Verification items for the finished model (mm, model axes). Face numbers are marked on the shaded views. A direction names the side the tool comes from. Round coordinates to 2 decimals unless told otherwise and drop trailing zeros. Order: outer loops, then holes, each group sorted by start corner. A loop starts at its lowest first (then second) coordinate and runs counter-clockwise, first axis right, second up. Notation, with made-up numbers: (-16, 6.5) -> (31, 6.5) arc R26 cw to (31, 26.5) -> close; hole circle Ø11 at (-7, 47). An arc over 180 degrees is marked (long way). Put each result on its own line as item: value.
Autodesk Inventor part; units mm, degrees
ref_plane "YZ Plane" through (0, 0, 0) normal (1, 0, 0) x (0, 1, 0)
ref_plane "XZ Plane" through (0, 0, 0) normal (0, 1, 0) x (-1, 0, 0)
ref_plane "XY Plane" through (0, 0, 0) normal (0, 0, 1) x (1, 0, 0)
sketch "Sketch1" plane through (0, 0, 0) normal (1, 0, 0) x (0, 1, 0)
  line L0 (-11, 0) -> (11, 0)
  line L1 (13, -8.587477) -> (0, -8.587477)
  line L2 (0, -8.587477) -> (0, 9)
  line L3 (0, 9) -> (4, 9)
  line L4 (4, 9) -> (11, 0) construction
  line L5 (4, 9) -> (13, 7)
  line L6 (13, 7) -> (13, 2)
  line L7 (13, 2) -> (13, 0)
  line L8 (4, 9) -> (0, 9)
  line L9 (0, 9) -> (0, 23)
  line L10 (0, 23) -> (4, 23)
  line L11 (4, 23) -> (4, 9)
  line L12 (13, -8.587477) -> (13, 0)
  point P0 (0, 0)
  dimension "d12" = 4
  dimension "d13" = 0
  dimension "d15" = 13
  dimension "d16" = 0
  dimension "d17" = 2
  dimension "d19" = 5
  dimension "d20" = 14
revolve "Revolution1" add sketch "Sketch1" angle 360 about axis through (0, 0, -8.587477) along (0, 0, 1)
sketch "Sketch4" plane through (0, 0, 23) normal (0, 0, 1) x (1, 0, 0)
  circle A0 centre (0, 0) radius 1.479649
  circle A1 centre (0, 0) radius 4
  circle A2 centre (0, 0) radius 3.25
  point P0 (0, 0)
  dimension "d21" = 6.5
extrude "Extrusion2" cut sketch "Sketch4" against normal through all contours A0 | A2
sketch "Sketch5" plane through (0, 0, -8.587477) normal (0, 0, -1) x (-1, 0, 0)
  circle A0 centre (0, 0) radius 11.938351
  circle A1 centre (0, 0) radius 11.2
  circle A2 centre (0, 0) radius 11
  point P0 (0, 0)
  dimension "d28" = 0.2
sketch "Sketch5 outline for Extrusion3" plane through (0, 0, -8.587477) normal (0, 0, -1) x (-1, 0, 0)
  circle A0 centre (0, 0) radius 11.2
extrude "Extrusion3" cut sketch "Sketch5 outline for Extrusion3" against normal blind 12 draft -3
fillet "Fillet2" radius 2 4 edges at (0, -4, 9) (0, -13, 7) (10.5711, 0, 3.4125) (-3.25, 0, 3.4125)
properties part number "01_Connector_T"
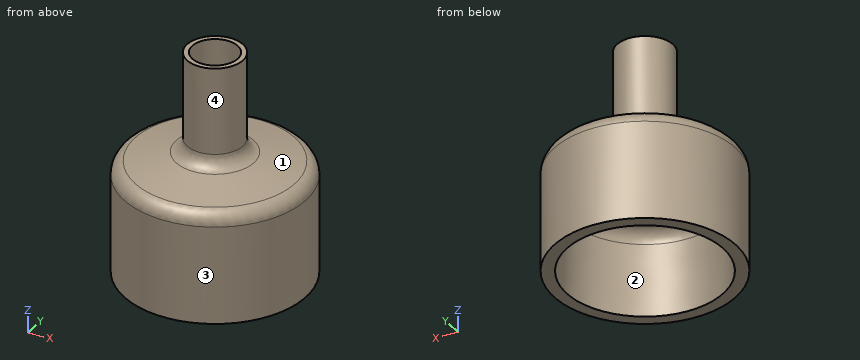
Item 1: Gauge pin test, flat ends, axial feed: pin 1 Ø8 at (x, y) = (0.5, -10) entering from -Z; pin 2 Ø4 at (x, y) = (-6, 3.5) entering from -Z; pin 3 Ø3 at (y, z) = (-2, -2) entering from -X; pin 4 Ø5 at (x, y) = (0, 0) entering from -Z. Record the tip position at first contact, or that the pin passes through.
Check sheet entries:
pin 1: stops at z = -8.59
pin 2: stops at z = 3.39
pin 3: stops at x = -12.99
pin 4: passes through
Item 2: Section check B-B on z = 1. Record the boundary of the cut face in (x, y), then the cut area to 3 significant figures.
Check sheet entries:
outline: circle Ø26 at (0, 0); hole circle Ø21.4 at (0, 0)
area: 171 mm^2
Item 3: Release check for a two-part mould opening along X. For the marked faces 1 and 2 record: +X half, -X half, draft (parallel to the pull), parting line (faces both ways), or undercut.
Check sheet entries:
face 1: parting line
face 2: undercut
Item 4: Material ranges on L1, parallel to Y at x = 0, z = 19.5; L2, parallel to X at y = 1.5, z = -3.5; L3, parallel to X at y = 1.75, z = 2.5, recorded low to high. Write a range as [from, to].
Check sheet entries:
L1: y = [-4, -3.25], [3.25, 4]
L2: x = [-12.91, -10.83], [10.83, 12.91]
L3: x = [-12.88, -10.2], [10.2, 12.88]
Item 5: Tool access check on the marked faces 3 and 4. Record the directions out of +Z, -Z, +X, -X, +Y, -Y that give a thin tool (end or side, any length) a straight path to the whole face; none if there is none.
Check sheet entries:
face 3: +Z, -Z
face 4: +Z
Item 6: Section check A-A on z = 17. Record the boundary of the cut face in (x, y), then the cut area to 3 significant figures.
Check sheet entries:
outline: circle Ø8 at (0, 0); hole circle Ø6.5 at (0, 0)
area: 17.1 mm^2
